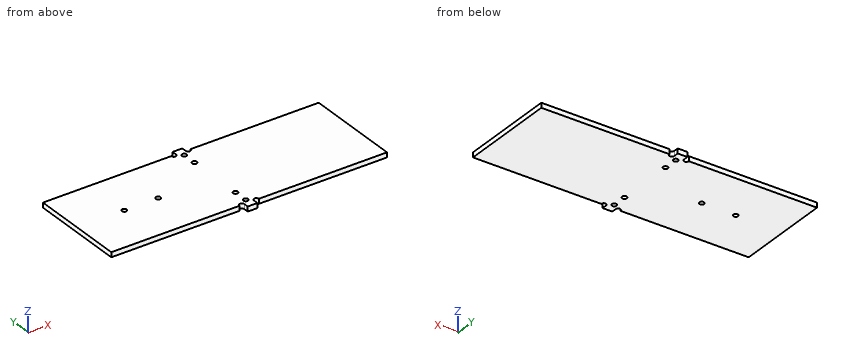
from build123d import *

# Parameters (mm, degrees)
SKETCH_1_R          = 1
EXTRUDE_1_DEPTH     = 2
SKETCH_2_R          = 1
CUT_EXTRUDE_1_DEPTH = 2


with BuildPart() as part:
    # 草圖1 → 填料-伸長1 (new body)
    with BuildSketch(Plane.XY):
        with BuildLine():
            Line((5.339530581, 31.894382022), (57.339530581, 31.894382022))
            Line((57.339530581, 31.894382022), (58.339530581, 31.894382022))
            Line((58.339530581, 31.894382022), (58.339530581, 30.894382022))
            Line((58.339530581, 30.894382022), (58.339530581, -7.105617978))
            Line((58.339530581, -7.105617978), (58.339530581, -8.105617978))
            Line((58.339530581, -8.105617978), (57.339530581, -8.105617978))
            Line((57.339530581, -8.105617978), (5.339530581, -8.105617978))
            ThreePointArc((5.339530581, -8.105617978), (4.339530581, -7.105617978), (3.339530581, -8.105617978))
            Line((3.339530581, -8.105617978), (3.339530581, -10.105617978))
            Line((3.339530581, -10.105617978), (-0.660469419, -10.105617978))
            Line((-0.660469419, -10.105617978), (-0.660469419, -8.105617978))
            ThreePointArc((-0.660469419, -8.105617978), (-1.660469419, -7.105617978), (-2.660469419, -8.105617978))
            Line((-2.660469419, -8.105617978), (-54.660469419, -8.105617978))
            Line((-54.660469419, -8.105617978), (-55.660469419, -8.105617978))
            Line((-55.660469419, -8.105617978), (-55.660469419, -7.105617978))
            Line((-55.660469419, -7.105617978), (-55.660469419, 30.894382022))
            Line((-55.660469419, 30.894382022), (-55.660469419, 31.894382022))
            Line((-55.660469419, 31.894382022), (-54.660469419, 31.894382022))
            Line((-54.660469419, 31.894382022), (-2.660469419, 31.894382022))
            ThreePointArc((-2.660469419, 31.894382022), (-1.660469419, 30.894382022), (-0.660469419, 31.894382022))
            Line((-0.660469419, 31.894382022), (-0.660469419, 33.894382022))
            Line((-0.660469419, 33.894382022), (3.339530581, 33.894382022))
            Line((3.339530581, 33.894382022), (3.339530581, 31.894382022))
            ThreePointArc((3.339530581, 31.894382022), (4.339530581, 30.894382022), (5.339530581, 31.894382022))
        make_face()
        with Locations((1.339530581, -6.105617978)):
            Circle(SKETCH_1_R, mode=Mode.SUBTRACT)
        with Locations((1.339530581, 29.894382022)):
            Circle(SKETCH_1_R, mode=Mode.SUBTRACT)
    extrude(amount=EXTRUDE_1_DEPTH)

    # 草圖2 → 除料-伸長1 (cut)
    with BuildSketch(Plane.XY.offset(2)):
        with Locations((1.339530581, 23.894382022)):
            Circle(SKETCH_2_R)
        with Locations((1.339530581, -0.105617978)):
            Circle(SKETCH_2_R)
        with Locations((-36.172114849, 11.894382022)):
            Circle(SKETCH_2_R)
        with Locations((-22.148823989, 11.894382022)):
            Circle(SKETCH_2_R)
    extrude(amount=-CUT_EXTRUDE_1_DEPTH, mode=Mode.SUBTRACT)


solid = part.part
Work out the finished part from the listing and answer in its coordinate system (mm). Give positions to 0.01 mm unless a question says otherwise; leave off trailing zeros. Loops run counter-clockwise (first coordinate to the right, second up) from the corner with the lowest first, then second, coordinate; pieces in that order, holes last. Notation, with made-up numbers: (-13.75, 83) -> (-9.75, 83) arc R16 cw to (-9.75, 103) -> close; hole circle Ø9 at (-3, -34). An arc over 180 degrees is marked (long way). Use a Markdown table: item, result. Add a question column.
1. Section B-B on x = -12 is taken. Determine the outline of the cut face in (y, z).
2. Flat-ended cylindrical pins translate along their axes: pin 1 Ø0.6 at (x, z) = (-35.5, 1.5) entering from +Y; pin 2 Ø1.6 at (x, y) = (1.34, -0.11) entering from +Z; pin 3 Ø1 at (y, z) = (33, 0.5) entering from +X; pin 4 Ø1 at (x, z) = (-16.5, 1.5) entering from -Y. Find the tip coordinate at first contact, or state that the pin passes through.
3. Find the intervals of material crossed by probe 1 along Y at (x, z) = (-9.5, 0.85); probe 2 along X at (y, z) = (32, 0.9); probe 3 along X at (y, z) = (-0.5, 1.2), in increasing order.
4. Section A-A on z = 0.8 is taken. Determine the outline of the cut face in (x, y), and give its area (3 significant figures).
Results below:
| question | item | result |
|---|---|---|
| 1 | outline | (-8.11, 0) -> (31.89, 0) -> (31.89, 2) -> (-8.11, 2) -> close |
| 2 | pin 1 | stops at y = 31.89 |
| 2 | pin 2 | passes through |
| 2 | pin 3 | stops at x = 3.34 |
| 2 | pin 4 | stops at y = -8.11 |
| 3 | probe 1 | y = -8.11 to 31.89 |
| 3 | probe 2 | x = -0.66 to 3.34 |
| 3 | probe 3 | x = -55.66 to 0.42, 2.26 to 58.34 |
| 4 | outline | (-55.66, -8.11) -> (-2.66, -8.11) arc R1 cw to (-0.66, -8.11) -> (-0.66, -10.11) -> (3.34, -10.11) -> (3.34, -8.11) arc R1 cw to (5.34, -8.11) -> (58.34, -8.11) -> (58.34, 31.89) -> (5.34, 31.89) arc R1 cw to (3.34, 31.89) -> (3.34, 33.89) -> (-0.66, 33.89) -> (-0.66, 31.89) arc R1 cw to (-2.66, 31.89) -> (-55.66, 31.89) -> close; hole circle Ø2 at (-36.17, 11.89); hole circle Ø2 at (-22.15, 11.89); hole circle Ø2 at (1.34, -6.11); hole circle Ø2 at (1.34, -0.11); hole circle Ø2 at (1.34, 23.89); hole circle Ø2 at (1.34, 29.89) |
| 4 | area | 4,550 mm^2 |
